CAD build for the part. Positions are in the model's coordinates, mm. A direction names the side the tool comes from. Give positions to 0.01 mm unless a question says otherwise; leave off trailing zeros. Write each loop counter-clockwise with the first axis right and the second up, starting at its lowest first coordinate (ties: lowest second). Pieces come first, ordered by that corner, then holes. Notation, with made-up numbers: (50.5, 15) - (60.5, 15) arc R25 cw to (60.5, 50) - close; hole circle Ø1 at (30.25, 36.25). An arc over 180 degrees is marked (long way). Write item = value, one per line. Start each with the question number.
```python
from build123d import *

# Parameters (mm, degrees)
SKETCH1_R           = 2
BOSS_EXTRUDE1_DEPTH = 2


with BuildPart() as part:
    # Sketch1 → Boss-Extrude1 (new, symmetric)
    with BuildSketch(Plane(origin=(0, 0, 0), x_dir=(1, 0, 0), z_dir=(0, 1, 0))):
        Polygon((-20.075, -4.29), (20.075, -4.29), (31.213284153, -37.981235074), (38.808958551, -35.470113721), (25.664309991, 4.29), (20.075, 4.29), (-20.075, 4.29), (-25.664309991, 4.29), (-38.808958551, -35.470113721), (-31.213284153, -37.981235074), align=None)
        with Locations(Location((14.075, 0, 0), (0, 0, 270))):
            Circle(SKETCH1_R, mode=Mode.SUBTRACT)
        with Locations(Location((-14.075, 0, 0), (0, 0, 90))):
            Circle(SKETCH1_R, mode=Mode.SUBTRACT)
        with Locations(Location((-32.5, -29.13, 0), (0, 0, 270))):
            Circle(SKETCH1_R, mode=Mode.SUBTRACT)
        with Locations(Location((32.5, -29.13, 0), (0, 0, 90))):
            Circle(SKETCH1_R, mode=Mode.SUBTRACT)
    extrude(amount=BOSS_EXTRUDE1_DEPTH, both=True)


solid = part.part
```
1. Cut at A-A (x = 32.5). Give the cut face in (y, z).
2. Cut at C-C (y = -1.05). Give the cut face in (x, z) (3 decimals), then the cut area to 3 significant figures.
3. Wall check: line 1 along Z through (x, y) = (-14, -0.65); line 2 along X through (y, z) = (-0.55, 0) (3 decimals); line 3 along X through (y, z) = (-0.2, 29.13). Give the ranges that are in metal, low to high.
4. Tool access for faces 4 (the flat face through (-25.72, 0.03, 21.37)), 5 (the cylindrical face through (15.76, -0.03, 1.08)): list every direction of +Z, -Z, +X, -X, +Y, -Y with a clear straight run to the whole face (end or side of a thin tool).
5. Cut at B-B (z = 7). Give the cut face in (x, y), then the cut area to 3 significant figures.
6. Cut at D-D (z = 29.13). Give the cut face in (x, y), then the cut area to 3 significant figures.
7. Mould opens along X. For faces 1 (the flat face through (32.33, 0.03, 15.87)), 2 (the cylindrical face through (-34.452, -0.028, 28.696)), 3 (the flat face through (0, 0, -4.29)) say: +X half, -X half, draft (parallel to the pull), parting line (faces both ways), or undercut.
8. Pin check, flat tip, straight feed: pin 1 Ø3.5 at (x, z) = (32.5, 29.13) entering from +Y. Stop position of the tip, or through.
Output:
q1.outline = (-2, 16.39) - (2, 16.39) - (2, 27.13) - (-2, 27.13) - close; (-2, 31.13) - (2, 31.13) - (2, 37.56) - (-2, 37.56) - close
q2.outline = (-38.809, 35.47) - (-25.664, -4.29) - (25.664, -4.29) - (38.809, 35.47) - (31.213, 37.981) - (20.075, 4.29) - (-20.075, 4.29) - (-31.213, 37.981) - close; hole circle Ø4 at (-32.5, 29.13); hole circle Ø4 at (-14.075, 0); hole circle Ø4 at (14.075, 0); hole circle Ø4 at (32.5, 29.13)
q2.area = 961 mm2
q3.line_1 = -4.29 to -2, 2 to 4.29
q3.line_2 = -27.083 to -16.075, -12.075 to 12.075, 16.075 to 27.083
q3.line_3 = -36.71 to -34.5, -30.5 to -28.29, 28.29 to 30.5, 34.5 to 36.71
q4.face_4 = +Z, +Y, -Y
q4.face_5 = +Y, -Y
q5.outline = (-29.4, -2) - (-20.97, -2) - (-20.97, 2) - (-29.4, 2) - close; (20.97, -2) - (29.4, -2) - (29.4, 2) - (20.97, 2) - close
q5.area = 67.4 mm2
q6.outline = (-36.71, -2) - (-34.5, -2) - (-34.5, 2) - (-36.71, 2) - close; (-30.5, -2) - (-28.29, -2) - (-28.29, 2) - (-30.5, 2) - close; (28.29, -2) - (30.5, -2) - (30.5, 2) - (28.29, 2) - close; (34.5, -2) - (36.71, -2) - (36.71, 2) - (34.5, 2) - close
q6.area = 35.4 mm2
q7.face_1 = +X half
q7.face_2 = undercut
q7.face_3 = draft
q8.pin_1 = through
